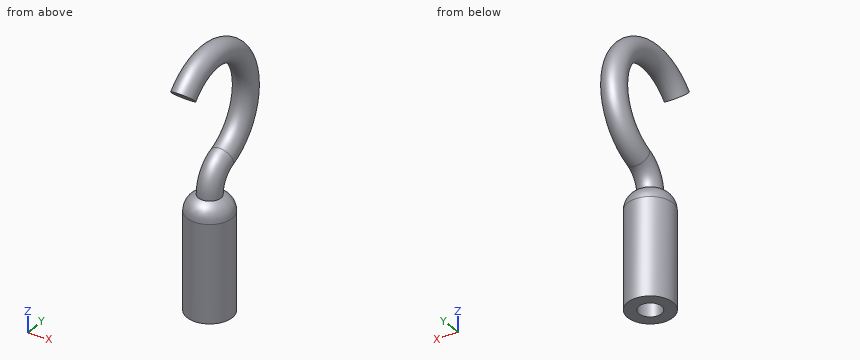
```python
from build123d import *

# Parameters (mm, degrees)
F0_R     = 4
F3_R     = 2
F6_R     = 2
F7_DEPTH = 10


# Not quite as in the source:
# - a fillet or chamfer that OpenCascade refuses, or shapes differently, is made with other operations: its cross-section is extruded or revolved along the edge and cut away or added


with BuildPart() as f2:
    # F2: sweep along a path in F1
    with BuildLine(Plane.YZ) as f2_path:
        Line((0, 0), (0, 20.0361318752))
    # F0 (on Top) → F2 (sweep)
    with BuildSketch(Plane.XY):
        Circle(F0_R)
    sweep(path=f2_path.line)

    # F4: sweep along a path in F1
    with BuildLine(Plane.YZ) as f4_path:
        ThreePointArc((0, 20.0361318752), (0.9181759559, 22.9238147652), (3.3354849893, 24.7509372561))
        ThreePointArc((3.3354849893, 24.7509372561), (8.2388991441, 39.4795133809), (-7.2441254742, 40.5977144837))
    # F3 (on face) → F4 (sweep)
    with BuildSketch(Plane.XY.offset(20.0361318752)):
        Circle(F3_R)
    sweep(path=f4_path.line)

    # F5: fillet of radius 3 on 1 edges, made by hand

    # F5_s1 → F5_t2 (revolve, cut)
    with BuildSketch(Plane.XZ):
        with BuildLine():
            ThreePointArc((4, 17.2077047505), (3.4494897428, 18.939755558), (2, 20.0361318752))
            Line((2, 20.0361318752), (2.02, 20.0927004177))
            ThreePointArc((2.02, 20.0927004177), (3, 20.0961318752), (4, 20.0961318752))
            Line((4, 20.0961318752), (4.06, 20.0361318752))
            Line((4.06, 20.0361318752), (4.06, 17.2077047505))
            Line((4.06, 17.2077047505), (4, 17.2077047505))
        make_face()
    revolve(axis=Axis((0, 0, 20.0361318752), (0, 0, 1)), mode=Mode.SUBTRACT)

    # F6 (on face) → F7 (cut)
    with BuildSketch(Plane(origin=(0, 0, 0), x_dir=(1, 0, 0), z_dir=(0, 0, -1))):
        Circle(F6_R)
    extrude(amount=-F7_DEPTH, mode=Mode.SUBTRACT)


solid = f2.part
```
For this review, take the finished solid that the model builds, in its own axes (mm). Round coordinates to 2 decimals unless told otherwise and drop trailing zeros. Loops run counter-clockwise (first coordinate to the right, second up) from the corner with the lowest first, then second, coordinate; pieces in that order, holes last.
Q1. To check wall thickness, follow line 1 along Y through (x, z) = (0, 4.5); line 2 along Z through (x, y) = (-0.5, 5.25); line 3 along X through (y, z) = (4.25, 25). State the ranges of each line that lie inside material, in increasing order.
Result sheet:
line 1: y = -4 to -2, 2 to 4
line 2: z = 23.46 to 28.07, 39.97 to 44.58
line 3: x = -2 to 2
Q2. Insertion check: pin 1 Ø3 at (x, z) = (-0.5, 29) entering from -Y; pin 2 Ø3 at (x, y) = (-2.5, 0.5) entering from +Z; pin 3 Ø1 at (x, y) = (-0.5, -4) entering from +Z. Each pin has a flat end and moves straight along its axis. Give the tip position at first contact, or say it passes through.
Result sheet:
pin 1: stops at y = 4.46
pin 2: stops at z = 45.58
pin 3: stops at z = 45.27
Q3. Add section A-A on z = 16.5. Write out the cut boundary in (x, y).
Result sheet:
outline: circle Ø8 at (0, 0)
